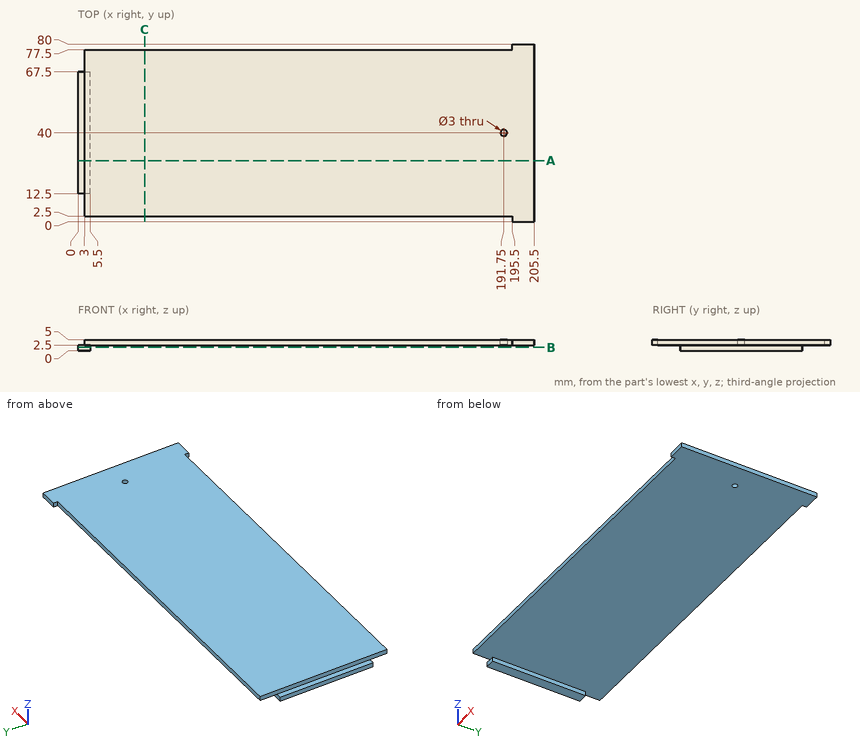
Can you work these out from the drawing? Everything is in mm from the part's minimum corner. Give positions to 0.01 mm unless a question says otherwise; leave off trailing zeros. Order: outer loops, then holes, each group sorted by start corner. A loop starts at its lowest first (then second) coordinate and runs counter-clockwise, first axis right, second up.
Item 1: I'm going to push flat-ended pins straight in: pin 1 (0.9 mm diameter, centred on x = 2, y = 48, fed in from +Z); pin 2 (2 mm diameter, centred on y = 51.5, z = 1, fed in from +X); pin 3 (24 mm diameter, centred on x = 88.5, y = 59, fed in from -Z). Where does each tip first touch, or does it pass through?
Item 2: If we section it at A-A, the plane y = 27.5: Write out the boundary of the cut face in (x, z), plus the area to 3 significant figures.
Item 3: If we section it at B-B, the plane z = 1.55: Write out the boundary of the cut face in (x, y).
Item 4: If we section it at C-C, the plane x = 30: Write out the boundary of the cut face in (y, z), plus the area to 4 significant figures.
Item 5: I need wall thicknesses on line 1 (Y direction, x = 191.75, z = 3.3); line 2 (X direction, y = 77, z = 2.75); line 3 (Z direction, x = 33, y = 32). Which ranges of each line are inside material? Lowest first, please.
Values:
1. pin 1: stops at z = 2.5
1. pin 2: stops at x = 5.5
1. pin 3: stops at z = 2.5
2. outline: (0, 0) - (5.5, 0) - (5.5, 2.5) - (205.5, 2.5) - (205.5, 5) - (3, 5) - (3, 2.5) - (0, 2.5) - close
2. area: 520 mm2
3. outline: (0, 12.5) - (5.5, 12.5) - (5.5, 67.5) - (0, 67.5) - close
4. outline: (2.5, 2.5) - (77.5, 2.5) - (77.5, 5) - (2.5, 5) - close
4. area: 187.5 mm2
5. line 1: y = 2.5 to 38.5, 41.5 to 77.5
5. line 2: x = 3 to 205.5
5. line 3: z = 2.5 to 5
